Geometry check sheet. Reference: the model listing, model coordinates, mm. A direction names the side the tool comes from. Coordinates: 2 decimals unless noted, no trailing zeros. Order: outer loops, then holes, each group sorted by start corner. A loop starts at its lowest first (then second) coordinate and runs counter-clockwise, first axis right, second up. Notation, with made-up numbers: M 6,53 L 53,53 A34 ccw 53,84 Z; hole C 68.5,-9.75 d8. An arc over 180 degrees is marked long. One line per item, written item: value. Start each with the question number.
1) Go/stop test with flat-tipped pins: P1, Ø2, axis at x = 22, z = 23, coming from the +Y side; P2, Ø2.5, axis at x = 25, y = 216, coming from the -Z side; P3, Ø4.5, axis at x = 24, y = 219, coming from the +Z side. Record where each tip stops, or that it passes through.
2) Sectioned sample at B-B, the plane z = -2. Enter the section's corners in (x, y) (3 decimals), then the cut area to 3 significant figures.
3) Sectioned sample at A-A, the plane y = 221.5. State how many separate pieces and enclosed holes the cut face has, then the cut area to 3 significant figures.
4) Access from +Z, -Z, +X, -X, +Y, -Y to the whole of each face (thin tool, end or side, straight path). Record for faces 5 (the flat face through (18, 6.756, 18)), 6 (the cylindrical face through (23.423, 237.136, -20.636)), 7 (the flat face through (-15.748, 220, -25)).
5) Thickness scan on L1, parallel to X at y = 3.75, z = -17.78 (3 decimals); L2, parallel to Y at x = -18.5, z = 19; L3, parallel to Y at x = 4.5, z = -19. Record the ranges inside material, lowest first. Write a range as from..to.
6) Draft check along Y on faces 1 (the flat face through (23, 235.204, 23)), 2 (the flat face through (-15.748, 221, 25)), 3 (the flat face through (-25, 220, 15.748)), 4 (the cylindrical face through (-25.49, 117.83, 25.4)). Enter one of: pulls with the +Y half, pulls with the -Y half, needs draft (parallel to the pull), parting line crosses it, or undercut.
```python
from build123d import *

# Parameters (mm, degrees)
BOSS_EXTRUDE1_DEPTH = 202.184
SKETCH2_R           = 2.1971
CUT_EXTRUDE1_DEPTH  = 6.7564
BOSS_EXTRUDE2_DEPTH = 36.83
CUT_EXTRUDE3_DEPTH  = 5.461
CIRPATTERN1_COUNT   = 4
SKETCH5_W           = 31.496
SKETCH5_H           = 5.08
CUT_EXTRUDE4_DEPTH  = 5.461
FILLET1_R           = 2.54
SKETCH6_R           = 2.2225
CUT_EXTRUDE5_DEPTH  = 3.81


with BuildPart() as part:
    # Sketch1 → Boss-Extrude1 (new body)
    with BuildSketch(Plane(origin=(0, 0, 0), x_dir=(1, 0, 0), z_dir=(0, 1, 0))):
        with BuildLine():
            Line((-20.955, -27.305), (20.955, -27.305))
            ThreePointArc((20.955, -27.305), (25.445128061, -25.445128061), (27.305, -20.955))
            Line((27.305, -20.955), (27.305, 20.955))
            ThreePointArc((27.305, 20.955), (25.445128061, 25.445128061), (20.955, 27.305))
            Line((20.955, 27.305), (-20.955, 27.305))
            ThreePointArc((-20.955, 27.305), (-25.445128061, 25.445128061), (-27.305, 20.955))
            Line((-27.305, 20.955), (-27.305, -20.955))
            ThreePointArc((-27.305, -20.955), (-25.445128061, -25.445128061), (-20.955, -27.305))
        make_face()
    extrude(amount=BOSS_EXTRUDE1_DEPTH)

    # Sketch2 → Cut-Extrude1 (cut)
    with BuildSketch(Plane.XZ):
        with Locations(Location((-17.78, 17.78, 0), (0, 0, 270))):
            Circle(SKETCH2_R)
        with Locations(Location((17.78, 17.78, 0), (0, 0, 90))):
            Circle(SKETCH2_R)
        with Locations(Location((17.78, -17.78, 0), (0, 0, 270))):
            Circle(SKETCH2_R)
        with Locations(Location((-17.78, -17.78, 0), (0, 0, 90))):
            Circle(SKETCH2_R)
    extrude(amount=-CUT_EXTRUDE1_DEPTH, mode=Mode.SUBTRACT)

    # Sketch3 → Boss-Extrude2 (add)
    with BuildSketch(Plane(origin=(0, 202.184, 0), x_dir=(1, 0, 0), z_dir=(0, 1, 0))):
        with BuildLine():
            Line((-27.305, 20.955), (-27.305, -20.955))
            ThreePointArc((-27.305, -20.955), (-25.445128061, -25.445128061), (-20.955, -27.305))
            Line((-20.955, -27.305), (20.955, -27.305))
            ThreePointArc((20.955, -27.305), (25.445128061, -25.445128061), (27.305, -20.955))
            Line((27.305, -20.955), (27.305, 20.955))
            ThreePointArc((27.305, 20.955), (25.445128061, 25.445128061), (20.955, 27.305))
            Line((20.955, 27.305), (-20.955, 27.305))
            ThreePointArc((-20.955, 27.305), (-25.445128061, 25.445128061), (-27.305, 20.955))
        make_face()
        Polygon((21.844, -18.288), (18.288, -21.844), (-18.288, -21.844), (-21.844, -18.288), (-21.844, 18.288), (-18.288, 21.844), (18.288, 21.844), (21.844, 18.288), align=None, mode=Mode.SUBTRACT)
    extrude(amount=BOSS_EXTRUDE2_DEPTH)

    # Sketch4 → Cut-Extrude3 (cut)
    with BuildSketch(Plane.ZY.offset(-21.844)):
        Polygon((-13.208, 236.474), (13.208, 236.474), (15.748, 233.934), (15.748, 207.264), (13.208, 204.724), (-13.208, 204.724), (-15.748, 207.264), (-15.748, 233.934), align=None)
    cut_extrude3 = extrude(amount=-CUT_EXTRUDE3_DEPTH, mode=Mode.SUBTRACT)

    # CirPattern1: Cut-Extrude3 ×4 about axis
    cirpattern1_axis = Axis((0, 0, 0), (0, 1, 0))
    for i in range(1, CIRPATTERN1_COUNT):
        add(cut_extrude3.rotate(cirpattern1_axis, i * 360 / CIRPATTERN1_COUNT), mode=Mode.SUBTRACT)

    # Sketch5 → Cut-Extrude4 (cut)
    with BuildSketch(Plane.ZY.offset(-21.844)):
        with Locations((0, 204.724)):
            Rectangle(SKETCH5_W, SKETCH5_H)
    extrude(amount=-CUT_EXTRUDE4_DEPTH, mode=Mode.SUBTRACT)

    # Fillet1
    fillet1_edges = [part.edges().sort_by_distance(p)[0] for p in [
        (24.5745, 202.184, 15.748),
        (24.5745, 202.184, -15.748),
    ]]
    fillet(fillet1_edges, radius=FILLET1_R)

    # Sketch6 → Cut-Extrude5 (cut)
    with BuildSketch(Plane(origin=(0, 239.014, 0), x_dir=(1, 0, 0), z_dir=(0, 1, 0))):
        with Locations(Location((22.75556403, -22.75556403, 0), (0, 0, 270))):
            Circle(SKETCH6_R)
        with Locations(Location((-22.75556403, -22.75556403, 0), (0, 0, 270))):
            Circle(SKETCH6_R)
        with Locations(Location((-22.75556403, 22.75556403, 0), (0, 0, 270))):
            Circle(SKETCH6_R)
        with Locations(Location((22.75556403, 22.75556403, 0), (0, 0, 270))):
            Circle(SKETCH6_R)
    extrude(amount=-CUT_EXTRUDE5_DEPTH, mode=Mode.SUBTRACT)


solid = part.part
```
Final values:
1. P1: stops at y = 235.2
1. P2: stops at z = -26.66
1. P3: stops at z = 27.26
2. outline: M -27.305,0 L 27.305,0 L 27.305,202.184 L -21.844,202.184 L -21.844,204.724 L -27.305,204.724 Z; M -27.305,236.474 L -21.844,236.474 L -21.844,239.014 L -27.305,239.014 Z; M 21.844,236.474 L 27.305,236.474 L 27.305,239.014 L 21.844,239.014 Z
2. area: 11,100 mm^2
3. separate pieces: 4
3. enclosed holes: 0
3. area: 376 mm^2
4. face 5: -Y
4. face 6: +Y
4. face 7: +Z, -Z
5. L1: x = -27.305..-19.977, -15.583..15.583, 19.977..27.305
5. L2: y = 6.76..202.18
5. L3: y = 0..202.18
6. face 1: pulls with the +Y half
6. face 2: undercut
6. face 3: undercut
6. face 4: needs draft
